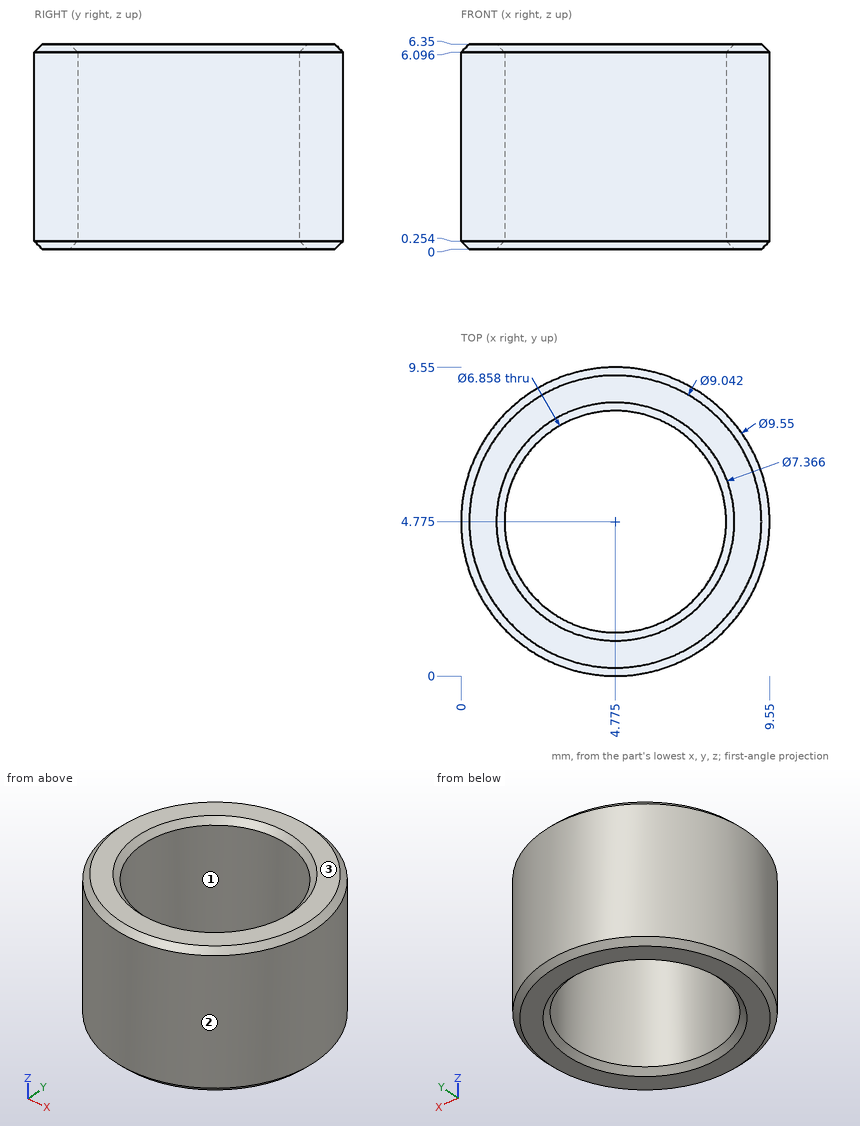
Print and shaded views of the part. All mm, measured from the part's lowest x, y and z. Round coordinates to 2 decimals unless told otherwise and drop trailing zeros.
Item 1: Probe L1, parallel to X at y = 6.25, z = 6.25 (1 decimal); L2, parallel to Y at x = 4.25, z = 1.75; L3, parallel to X at y = 2.25, z = 2 (1 decimal). List the from-to ranges inside material, lowest first.
Results:
L1: x = 0.4 to 1.5, 8 to 9.2
L2: y = 0.03 to 1.39, 8.16 to 9.52
L3: x = 0.7 to 2.5, 7.1 to 8.8
Item 2: Two-plate mould, pull along Y, no slides. Class the marked faces 1, 2 and 3: +Y half, -Y half, draft (parallel to the pull), parting line (faces both ways), or undercut.
Results:
face 1: undercut
face 2: parting line
face 3: draft
Item 3: Drop flat-ended pins along their axis: pin 1 Ø2 at (y, z) = (8.5, 4) entering from +X; pin 2 Ø2 at (x, y) = (3, 3) entering from +Z; pin 3 Ø2 at (x, z) = (8, 5) entering from +Y; pin 4 Ø3 at (x, y) = (5.5, 4) entering from +Z. Give the stop position or say it passes through.
Results:
pin 1: stops at x = 8.7
pin 2: stops at z = 6.18
pin 3: stops at y = 9
pin 4: passes through
